Model file for the job. Use its own axes, mm. A direction names the side the tool comes from. Coordinates: 2 decimals unless noted, no trailing zeros. Write each loop counter-clockwise with the first axis right and the second up, starting at its lowest first coordinate (ties: lowest second). Pieces come first, ordered by that corner, then holes. Notation, with made-up numbers: (25.5, 42.5) - (66.5, 42.5) arc R32 cw to (66.5, 69.5) - close; hole circle Ø4 at (16.25, -35). An arc over 180 degrees is marked (long way). Put each result on its own line as item: value. Start each with the question number.
1. Drop flat-ended pins along their axis: P1, Ø3, axis at x = -32, z = 25, coming from the -Y side; P2, Ø5, axis at y = -59, z = -7.5, coming from the -X side; P3, Ø5, axis at y = -61, z = -6.5, coming from the +X side; P4, Ø22, axis at x = 9, z = -5, coming from the -Y side. Give the stop position or say it passes through.
2. Saw through at D-D, the plane z = 26. Write the cut outline in (x, y).
3. Saw through at A-A, the plane z = -13. Write the cut outline in (x, y) (3 decimals).
4. Drill centre lines: L1, parallel to Y at x = -12, z = -12.5; L2, parallel to Y at x = -22.5, z = -7; L3, parallel to Z at x = 2, y = -92. Where is each one in solid material? Low to high. Write a range as from..to.
5. Saw through at C-C, the plane x = -2.5. Write the cut outline in (y, z).
6. Saw through at B-B, the plane y = 50.5. Write the cut outline in (x, z) (3 decimals), plus the area to 3 significant figures.
7. Which spindle directions (+Z, -Z, +X, -X, +Y, -Y) get a long thin tool onto all of the face, cutting with end or side? Do faces 5 (the face through (-1, -59, -17.272)), 6 (the face through (-30.185, 44, -10)), 7 (the face through (19.427, -59, -9)), 8 (the face through (1, 65.012, -10)). Say none if no direction does.
8. Pull direction Y, two halves, no side cores. Call faces 1 (the face through (28.517, -16, -10)), 2 (the face through (-1, 0, -10)), 3 (the face through (-1, -51.166, -9)), 4 (the face through (-1, -67.447, -9)): released by +Y, released by -Y, zero draft, split by the parting line, or undercut.
```python
from build123d import *

# Parameters (mm, degrees)
F1_DEPTH = 34.544
F2_W     = 40.292801
F2_H     = 16.280751
F3_DEPTH = 17.272
F4_W     = 62.371195
F4_H     = 41.358443
F4_W_2   = 57.368159
F4_H_2   = 31.046361
F5_DEPTH = 20.066


with BuildPart() as f1:
    # F0 (on Top) → F1 (new body)
    with BuildSketch(Plane.XY):
        Polygon((-42.372001, 77.851459), (-42.372001, -33.529375), (42.372001, -33.529375), (42.451348, -33.529375), (42.451348, 77.851459), (42.451348, 109.199524), (-42.372001, 109.199524), align=None)
        Polygon((42.372001, -33.529375), (-42.372001, -33.529375), (0, -106.919833), align=None)
    extrude(amount=F1_DEPTH)

    # F2 (on Top) → F3 (join)
    with BuildSketch(Plane.XY):
        with Locations((-0.719514, -59.306254)):
            Rectangle(F2_W, F2_H)
    extrude(amount=-F3_DEPTH)

    # F4 (on Top) → F5 (join)
    with BuildSketch(Plane.XY):
        with Locations((1.000606, 44.332735)):
            Rectangle(F4_W, F4_H)
        with Locations((-0.166768, -15.52318)):
            Rectangle(F4_W_2, F4_H_2)
    extrude(amount=-F5_DEPTH)


solid = f1.part
```
Final values:
1. P1: stops at y = -54.09
1. P2: stops at x = -20.87
1. P3: stops at x = 19.43
1. P4: stops at y = -106.92
2. outline: (-42.37, -33.53) - (0, -106.92) - (42.37, -33.53) - (42.45, -33.53) - (42.45, 109.2) - (-42.37, 109.2) - close
3. outline: (-30.185, 23.654) - (32.186, 23.654) - (32.186, 65.012) - (-30.185, 65.012) - close; (-28.851, -31.046) - (28.517, -31.046) - (28.517, 0) - (-28.851, 0) - close; (-20.866, -67.447) - (19.427, -67.447) - (19.427, -51.166) - (-20.866, -51.166) - close
4. L1: y = -67.45..-51.17, -31.05..0, 23.65..65.01
4. L2: y = -31.05..0, 23.65..65.01
4. L3: z = 0..34.54
5. outline: (-102.59, 0) - (-67.45, 0) - (-67.45, -17.27) - (-51.17, -17.27) - (-51.17, 0) - (-31.05, 0) - (-31.05, -20.07) - (0, -20.07) - (0, 0) - (23.65, 0) - (23.65, -20.07) - (65.01, -20.07) - (65.01, 0) - (109.2, 0) - (109.2, 34.54) - (-102.59, 34.54) - close
6. outline: (-42.372, 0) - (-30.185, 0) - (-30.185, -20.066) - (32.186, -20.066) - (32.186, 0) - (42.451, 0) - (42.451, 34.544) - (-42.372, 34.544) - close
6. area: 4,180 mm²
7. face 5: -Z, +X, -X, -Y
7. face 6: -Z, -X, +Y, -Y
7. face 7: -Z, +X, -Y
7. face 8: -Z, +X, -X, +Y
8. face 1: zero draft
8. face 2: undercut
8. face 3: undercut
8. face 4: released by -Y
